Input: part model. Units: mm. Frame: model coordinates. Face numbers are marked on the shaded views. Give positions to 0.01 mm unless a question says otherwise; leave off trailing zeros. Loops run counter-clockwise (first coordinate to the right, second up) from the corner with the lowest first, then second, coordinate; pieces in that order, holes last. Notation, with made-up numbers: M 45,-19.75 L 94,-19.75 A34 cw 94,13.25 Z; hole C 44.5,66 d11. An arc over 180 degrees is marked long. Answer as a JSON object with one key per item and string values. Group by question number.
1) Ray query, L1, parallel to Y at x = 7.25, z = 23; L2, parallel to Y at x = 7, z = 4.5; L3, parallel to Y at x = 3.5, z = 14. Return the intervals inside material, ascending.
2) Section query B-B on y = 4.25. Return loops of the section in (x, z), plus the area to 3 significant figures.
3) First-contact query: P1, Ø1, axis at y = 5, z = 14.5, coming from the +X side; P2, Ø2, axis at y = -2, z = 6.5, coming from the -X side; P3, Ø2, axis at y = 7, z = 24, coming from the -X side. Flat tips, straight axial feed; report the tip coordinate or a pass-through.
4) Draft query along Y for the marked faces 1, 2, 3 and 4. Return one class per face: +Y half, -Y half, draft (parallel to the pull), parting line (faces both ways), or undercut.
5) Section query C-C on x = 4. Return loops of the section in (y, z).
from build123d import *

# Parameters (mm, degrees)
SKETCH1_R           = 11.15
BOSS_EXTRUDE1_DEPTH = 31.75
CUT_EXTRUDE4_DEPTH  = 36.450070522
FILLET2_R           = 1
FILLET4_R           = 1


with BuildPart() as part:
    # Sketch1 → Boss-Extrude1 (new body)
    with BuildSketch(Plane.XY):
        Circle(SKETCH1_R)
    extrude(amount=BOSS_EXTRUDE1_DEPTH)

    # Sketch2 → Cut-Extrude4 (cut, through all)
    with BuildSketch(Plane.XY):
        with BuildLine():
            Line((0, 6.5), (0, 9))
            ThreePointArc((0, 9), (-4.835696475, 7.590523012), (-8.156770083, 3.803564356))
            Line((-8.156770083, 3.803564356), (-5.891000616, 2.747018701))
            ThreePointArc((-5.891000616, 2.747018701), (-6.345924046, 1.406857491), (-6.5, 0))
            Line((-6.5, 0), (-9, 0))
            ThreePointArc((-9, 0), (-7.590523012, -4.835696475), (-3.803564356, -8.156770083))
            Line((-3.803564356, -8.156770083), (-2.747018701, -5.891000616))
            ThreePointArc((-2.747018701, -5.891000616), (-1.406857491, -6.345924046), (0, -6.5))
            Line((0, -6.5), (0, -9))
            ThreePointArc((0, -9), (4.835696475, -7.590523012), (8.156770083, -3.803564356))
            Line((8.156770083, -3.803564356), (5.891000616, -2.747018701))
            ThreePointArc((5.891000616, -2.747018701), (6.345924046, -1.406857491), (6.5, 0))
            Line((6.5, 0), (9, 0))
            ThreePointArc((9, 0), (7.590523012, 4.835696475), (3.803564356, 8.156770083))
            Line((3.803564356, 8.156770083), (2.747018701, 5.891000616))
            ThreePointArc((2.747018701, 5.891000616), (1.406857491, 6.345924046), (0, 6.5))
        make_face()
    extrude(amount=CUT_EXTRUDE4_DEPTH, mode=Mode.SUBTRACT)

    # Fillet2
    fillet2_edges = [part.edges().sort_by_distance(p)[0] for p in [
        (6.345924046, -1.406857491, 0),
        (5.891000616, -2.747018701, 15.875),
        (6.5, 0, 15.875),
        (1.406857491, 6.345924046, 0),
        (2.747018701, 5.891000616, 15.875),
        (0, 6.5, 15.875),
        (-6.345924046, 1.406857491, 0),
        (-5.891000616, 2.747018701, 15.875),
        (-6.5, 0, 15.875),
        (-1.406857491, -6.345924046, 0),
        (-2.747018701, -5.891000616, 15.875),
        (0, -6.5, 15.875),
        (6.345924046, -1.406857491, 31.75),
        (1.406857491, 6.345924046, 31.75),
        (-6.345924046, 1.406857491, 31.75),
        (-1.406857491, -6.345924046, 31.75),
    ]]
    fillet(fillet2_edges, radius=FILLET2_R)

    # Fillet4
    fillet4_edges = [part.edges().sort_by_distance(p)[0] for p in [
        (9, 0, 15.875),
        (3.803564356, 8.156770083, 15.875),
        (0, 9, 15.875),
        (-8.156770083, 3.803564356, 15.875),
        (-9, 0, 15.875),
        (-3.803564356, -8.156770083, 15.875),
        (0, -9, 15.875),
        (8.156770083, -3.803564356, 15.875),
    ]]
    fillet(fillet4_edges, radius=FILLET4_R)


solid = part.part
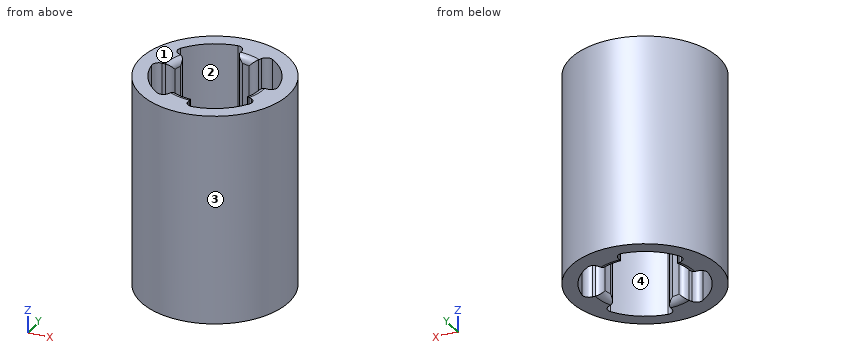
Output:
{
 "1": {"L1": "y = -8.47 to -5.33, -3.38 to -0.02, 5.33 to 8.47", "L2": "y = -8.68 to -5.66, -3.26 to -0.1, 5.66 to 8.68", "L3": "y = -10.59 to -8.29, 7.42 to 10.59"},
 "2": {"outline": "M -10.31,0 L -7.77,0 L -7.77,31.75 L -10.31,31.75 Z; M 7.93,0 L 10.31,0 L 10.31,31.75 L 7.93,31.75 Z", "area": "156 mm^2"},
 "3": {"P1": "stops at x = 10.2", "P2": "stops at x = -11.11", "P3": "stops at x = -9.4"},
 "4": {"face 1": "draft", "face 2": "undercut", "face 3": "parting line", "face 4": "undercut"},
 "5": {"outline": "M -10.41,0 L -8.06,0 L -8.06,31.75 L -10.41,31.75 Z; M 7.74,0 L 10.41,0 L 10.41,31.75 L 7.74,31.75 Z"}
}
